Check sheet for the modelled part. Datum: model origin and axes. Units: mm. A direction names the side the tool comes from. Round coordinates to 2 decimals unless told otherwise and drop trailing zeros. Order: outer loops, then holes, each group sorted by start corner. A loop starts at its lowest first (then second) coordinate and runs counter-clockwise, first axis right, second up.
Q1. Mould release check, pull along X, two halves, no side actions. Record for faces 1 (the flat face through (3, 17.732, 0)), 2 (the conical face through (0, 0, 0)), 3 (the flat face through (-0.95, 17, 0)): +X half, -X half, draft (parallel to the pull), parting line (faces both ways), or undercut.
Q2. Set-up check for faces 4 (the flat face through (0, 16.132, 0)), 5 (the flat face through (-3, 17.732, 0)), 6 (the cylindrical face through (-3, 8, 0)): record each of +Z, -Z, +X, -X, +Y, -Y from which the full face is reachable in a straight line by a thin tool's end or side.
Q3. Depth check by flat-ended pin: P1, Ø5, axis at x = 2.5, z = -3, coming from the -Y side; P2, Ø1.8, axis at y = 17, z = -0.5, coming from the +X side; P3, Ø1.5, axis at y = 9, z = 1, coming from the -X side; P4, Ø1.8, axis at y = 17, z = 2.5, coming from the -X side. Enter the tip coordinate at first touch or a pass-through.
Q4. Scan lines: probe 1 along X at (y, z) = (17, 0.5); probe 2 along X at (y, z) = (16.5, -3.75); probe 3 along Y at (x, z) = (2, 2.5). Record each from-to range of solid material in increasing order.
Q5. Cross-section at A-A on y = 6. Record the cut outline in (x, z).
from build123d import *

# Parameters (mm, degrees)
SKETCH2_W               = 1.9
SKETCH2_H               = 1.6
CUT_EXTRUDE1_DEPTH      = 6.45
CUT_EXTRUDE1_DEPTH_BACK = 6.45


with BuildPart() as part:
    # Sketch1 → Revolve1 (revolve)
    with BuildSketch(Plane.XY):
        Polygon((0, 0), (0, 17.732050808), (5.45, 17.732050808), (3, 15.282050808), (3, 1.732050808), align=None)
    revolve(axis=Axis((0, 0, 0), (0, 1, 0)))

    # Sketch2 → Cut-Extrude1 (cut, two sides)
    with BuildSketch(Plane.XY) as cut_extrude1_sk:
        with Locations((0, 16.932050808)):
            Rectangle(SKETCH2_W, SKETCH2_H)
    extrude(amount=CUT_EXTRUDE1_DEPTH, mode=Mode.SUBTRACT)
    extrude(cut_extrude1_sk.sketch, amount=-CUT_EXTRUDE1_DEPTH_BACK, mode=Mode.SUBTRACT)


solid = part.part
Results found:
1. face 1: draft
1. face 2: parting line
1. face 3: undercut
2. face 4: +Z, -Z, +Y
2. face 5: +Z, -Z, +X, -X, +Y
2. face 6: -Y
3. P1: stops at y = 0.81
3. P2: stops at x = 5.45
3. P3: stops at x = -2.99
3. P4: stops at x = -5.08
4. probe 1: x = -4.69 to -0.95, 0.95 to 4.69
4. probe 2: x = -1.93 to -0.95, 0.95 to 1.93
4. probe 3: y = 15.48 to 17.73
5. outline: circle Ø6 at (0, 0)
